Read the model definition and answer for the solid it produces. Units are mm, in the model's axes. Face numbers are marked on the shaded views. Round coordinates to 2 decimals unless told otherwise and drop trailing zeros. Write each loop counter-clockwise with the first axis right and the second up, starting at its lowest first coordinate (ties: lowest second). Pieces come first, ordered by that corner, then holes. Notation, with made-up numbers: (50, 5.5) - (105, 5.5) arc R15 ccw to (105, 17.5) - close; hole circle Ø11 at (77.5, 40.5). An arc over 180 degrees is marked (long way). Answer as CSV lines item,"result". Start each with the question number.
1) Find section C-C on z = 40.5. Determine the outline of the cut face in (x, y), then the cut area to 3 significant figures.
2) Find section B-B on z = 24. Determine the outline of the cut face in (x, y), then the cut area to 3 significant figures.
3) For a pull along Z with two mould halves and no side action, classify the marked faces 1, 2 and 3 as +Z half, -Z half, draft (parallel to the pull), parting line (faces both ways), or undercut.
4) Consider line 1 along Y through (x, z) = (0, 1); line 2 along Z through (x, y) = (20, -8.5); line 3 along X through (y, z) = (12, 16.5). Determine where each line is inside the solid, lowest interval first.
5) Each of these flat-tipped pins is pushed along its axis until it touches: pin 1 (10 mm diameter, centred on x = -11.5, z = 38.5, fed in from -Y); pin 2 (1 mm diameter, centred on x = -16, z = 0.5, fed in from +Y); pin 3 (2 mm diameter, centred on x = -0.5, z = 0.5, fed in from +Y). Where does it stop, or does it pass through?
from build123d import *

# Parameters (mm, degrees)
F1_DEPTH = 2
F2_R     = 1
F3_R     = 9
F4_DEPTH = 2
F8_W     = 24
F8_H     = 2
F9_DEPTH = 10


with BuildPart() as f1:
    # F0 (on Top) → F1 (new body)
    with BuildSketch(Plane.XY):
        Polygon((-12, 8.716256), (-24, 8.716256), (-24, -19.283744), (17, -19.283744), (17, 8.716256), (12, 8.716256), (12, 29.716256), (-12, 29.716256), align=None)
    extrude(amount=F1_DEPTH)

    # F2
    f2_edges = [f1.edges().sort_by_distance(p)[0] for p in [
        (-24, 8.716256, 1),
        (-12, 29.716256, 1),
        (12, 29.716256, 1),
        (17, 8.716256, 1),
        (17, -19.283744, 1),
        (-24, -19.283744, 1),
    ]]
    fillet(f2_edges, radius=F2_R)

    # F3 (on face) → F4 (cut, through all)
    with BuildSketch(Plane.XY.offset(2)):
        with Locations((0, 18.716256)):
            Circle(F3_R)
    extrude(amount=-F4_DEPTH, mode=Mode.SUBTRACT)

    # F5 (on Right) → F7 (revolve)
    with BuildSketch(Plane.YZ):
        Polygon((36.509466, 52), (27.693117, 2), (29.216256, 2), (38.032605, 52), align=None)
    revolve(axis=Axis((0, 18.716256, 10.515208), (0, 0, 1)))

    # F8 (on face) → F9 (join)
    with BuildSketch(Plane.YZ.offset(17)):
        with Locations((-5.283744, 1)):
            Rectangle(F8_W, F8_H)
    extrude(amount=F9_DEPTH)


solid = f1.part
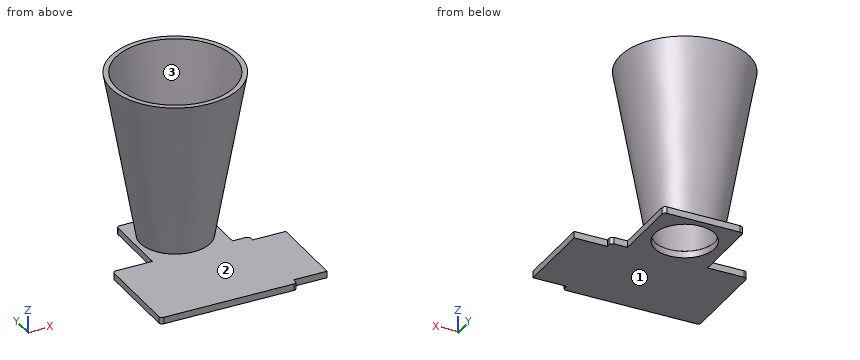
Check values:
1,outline,"circle Ø34.58 at (0, 18.72); hole circle Ø31.53 at (0, 18.72)"
1,area,"158 mm^2"
2,outline,"circle Ø28.76 at (0, 18.72); hole circle Ø25.71 at (0, 18.72)"
2,area,"130 mm^2"
3,face 1,"-Z half"
3,face 2,"undercut"
3,face 3,"+Z half"
4,line 1,"y = -19.28 to 9.72, 27.72 to 29.72"
4,line 2,"z = 0 to 2"
4,line 3,"x = -11.2 to -9.38, 9.38 to 11.2"
5,pin 1,"stops at y = 2.87"
5,pin 2,"stops at y = 8.72"
5,pin 3,"stops at y = 29.72"
